Can you work these out from the drawing? Everything is in mm from the part's minimum corner. A direction names the side the tool comes from. Coordinates: 2 decimals unless noted, no trailing zeros. Order: outer loops, then holes, each group sorted by start corner. A loop starts at its lowest first (then second) coordinate and runs counter-clockwise, first axis right, second up. Notation, with made-up numbers: (-2, 69.5) - (35, 69.5) arc R18 ccw to (35, 84.5) - close; hole circle Ø2 at (-3, 12). An arc over 180 degrees is marked (long way). Use a Markdown table: item, result. Add a question column.
(1) I want a section at B-B (z = 33.5). List the corners of the cut face in (x, y) for me.
(2) If I drill on L1, parallel to X at y = 3.35, z = 9.95; L2, parallel to Z at x = 40.5, y = 36; L3, parallel to X at y = 3, z = 33, over which ranges is the centre line in solid material (lowest first)? Write a range as [from, to].
(3) I want a section at C-C (y = 4). List the corners of the cut face in (x, z) for me, and give its area (3 significant figures).
(4) For pin 1 Ø17 at (y, z) = (42, 31) entering from -X; pin 2 Ø3 at (x, z) = (4.95, 9.95) entering from -Y; pin 3 Ø17 at (x, z) = (29, 22.5) entering from +Y, each with a flat end and sliding along its axis, tell me the tip position at first contact or that it passes through.
(5) I want a section at D-D (z = 9.95). List the corners of the cut face in (x, y) for me, and give its area (3 significant figures).
(6) I want a section at A-A (x = 52.05). List the corners of the cut face in (y, z) for me.
(7) We'd pull the mould along Z, two halves only. Please class the marked faces 3, 4 and 5: pulls with the +Z half, pulls with the -Z half, needs draft (parallel to the pull), parting line crosses it, or undercut.
(8) On a 3-axis mill with a long thin cutter (end or side, diameter ignored), from which of +Z, -Z, +X, -X, +Y, -Y can I reach the whole of each face in a straight line? I mean the marked faces 1 and 2. Say none if no direction works.
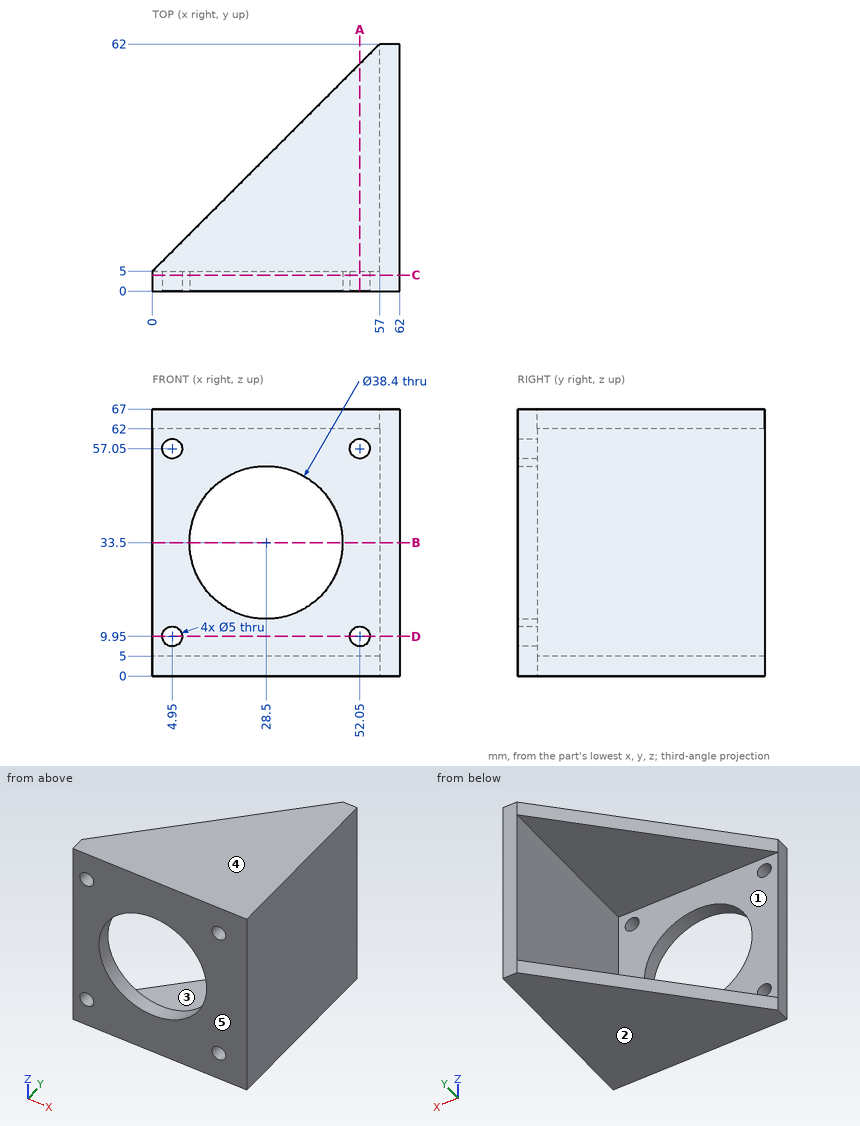
Answers follow:
| question | item | result |
|---|---|---|
| 1 | outline | (0, 0) - (9.3, 0) - (9.3, 5) - (0, 5) - close; (47.7, 0) - (62, 0) - (62, 62) - (57, 62) - (57, 5) - (47.7, 5) - close |
| 2 | L1 | x = [0, 2.45], [7.45, 49.55], [54.55, 62] |
| 2 | L2 | z = [0, 5], [62, 67] |
| 2 | L3 | x = [0, 9.31], [47.69, 62] |
| 3 | outline | (0, 0) - (62, 0) - (62, 67) - (0, 67) - close; hole circle Ø5 at (4.95, 9.95); hole circle Ø5 at (4.95, 57.05); hole circle Ø38.4 at (28.5, 33.5); hole circle Ø5 at (52.05, 9.95); hole circle Ø5 at (52.05, 57.05) |
| 3 | area | 2,920 mm² |
| 4 | pin 1 | stops at x = 57 |
| 4 | pin 2 | passes through |
| 4 | pin 3 | stops at y = 5 |
| 5 | outline | (0, 0) - (2.45, 0) - (2.45, 5) - (0, 5) - close; (7.45, 0) - (49.55, 0) - (49.55, 5) - (7.45, 5) - close; (54.55, 0) - (62, 0) - (62, 62) - (57, 62) - (57, 5) - (54.55, 5) - close |
| 5 | area | 545 mm² |
| 6 | outline | (0, 0) - (57.05, 0) - (57.05, 5) - (5, 5) - (5, 7.45) - (0, 7.45) - close; (0, 12.45) - (5, 12.45) - (5, 54.55) - (0, 54.55) - close; (0, 59.55) - (5, 59.55) - (5, 62) - (57.05, 62) - (57.05, 67) - (0, 67) - close |
| 7 | face 3 | undercut |
| 7 | face 4 | pulls with the +Z half |
| 7 | face 5 | needs draft |
| 8 | face 1 | -X, +Y |
| 8 | face 2 | -Z, +X, -X, +Y, -Y |
